Here's how the part is built. I have some questions about the finished solid (model axes, mm). A direction names the side the tool comes from. Round coordinates to 2 decimals unless told otherwise and drop trailing zeros. Write each loop counter-clockwise with the first axis right and the second up, starting at its lowest first coordinate (ties: lowest second). Pieces come first, ordered by that corner, then holes. Notation, with made-up numbers: M 41.5,38.5 L 65.5,38.5 A21 cw 65.5,42.5 Z; hole C 79,89.25 d4. An arc over 180 degrees is marked long. Write item = value, one per line. Start each with the question number.
(1) I want a section at C-C (z = -33). List the corners of the cut face in (x, y) for me.
(2) On a 3-axis mill with a long thin cutter (end or side, diameter ignored), from which of +Z, -Z, +X, -X, +Y, -Y can I reach the whole of each face in a straight line? I mean faces 1 (the flat face through (140, 2, -77)), 2 (the flat face through (98, 0, -24)), 3 (the flat face through (146.216, 1.972, 46.336)), 4 (the flat face through (160, 2, -73)), 5 (the flat face through (49.06, 1.97, 44.46)). Say none if no direction works.
(3) I want a section at D-D (y = 2.15). Give the number of separate pieces and of enclosed holes in the cut face, and give its area (3 significant figures).
(4) If we mould it in two halves opening along X, with no side actions, what happens to faces 6 (the flat face through (-4, 2, -9)), 7 (the flat face through (199, 2, 0)), 8 (the flat face through (190, 2, -75)), 9 (the cylindrical face through (100, 2, 62))? For each: released by +X, released by -X, zero draft, split by the parting line, or undercut.
(5) I want a section at A-A (z = -56). List the corners of the cut face in (x, y) for me, and give its area (3 significant figures).
(6) I want a section at B-B (x = 63). List the corners of the cut face in (y, z) for me.
(7) I need wall thicknesses on line 1 along X through (y, z) = (1.05, -33); line 2 along X through (y, z) = (2.8, -11.5); line 3 along X through (y, z) = (0.4, -53.5). Which ranges of each line are inside material? Lowest first, please.
(8) Will these pins go through, and if not, where does the flat tip stop? pin 1 Ø2 at (y, z) = (1.5, -74.5) entering from +X; pin 2 Ø1.5 at (x, y) = (152.5, 1) entering from -Z; pin 3 Ø2.5 at (x, z) = (137, -33) entering from -Y; pin 4 Ø1.5 at (x, y) = (97.5, 0.5) entering from -Z.
```python
from build123d import *

# Parameters (mm, degrees)
SKICA1_W                = 4
SKICA1_H                = 15
SKICA1_R                = 2.25
P_IDAT_VYSUNUT_M1_DEPTH = 4


with BuildPart() as part:
    # Skica1 → Přidat vysunutím1 (new body)
    with BuildSketch(Plane(origin=(0, 0, 0), x_dir=(1, 0, 0), z_dir=(0, 1, 0))):
        with BuildLine():
            ThreePointArc((10.915770195, 0), (25.940686176, -26.499731394), (48.580654593, -46.881480444))
            Line((48.580654593, -46.881480444), (49.547625125, -41.975874672))
            Line((49.547625125, -41.975874672), (54.453230897, -42.942845204))
            Line((54.453230897, -42.942845204), (53.134056197, -49.635242551))
            ThreePointArc((53.134056197, -49.635242551), (64.622092485, -55.166907964), (76.747418364, -59.110354723))
            Line((76.747418364, -59.110354723), (78.981259757, -47.777697862))
            Line((78.981259757, -47.777697862), (83.886865529, -48.744668394))
            Line((83.886865529, -48.744668394), (81.627559896, -60.206509669))
            ThreePointArc((81.627559896, -60.206509669), (100, -62), (118.372440104, -60.206509669))
            Line((118.372440104, -60.206509669), (116.113134471, -48.744668394))
            Line((116.113134471, -48.744668394), (121.018740243, -47.777697862))
            Line((121.018740243, -47.777697862), (123.252581636, -59.110354723))
            ThreePointArc((123.252581636, -59.110354723), (135.377907515, -55.166907964), (146.865943803, -49.635242551))
            Line((146.865943803, -49.635242551), (145.546769103, -42.942845204))
            Line((145.546769103, -42.942845204), (150.452374875, -41.975874672))
            Line((150.452374875, -41.975874672), (151.419345407, -46.881480444))
            ThreePointArc((151.419345407, -46.881480444), (174.059313824, -26.499731394), (189.084229805, 0))
            Line((189.084229805, 0), (209, 0))
            Line((209, 0), (209, 53))
            Line((209, 53), (200, 53))
            Line((200, 53), (200, 73))
            Line((200, 73), (190, 73))
            Line((190, 73), (190, 77))
            Line((190, 77), (170, 77))
            Line((170, 77), (170, 73))
            Line((170, 73), (150, 73))
            Line((150, 73), (150, 77))
            Line((150, 77), (130, 77))
            Line((130, 77), (130, 73))
            Line((130, 73), (115, 73))
            Line((115, 73), (115, 53))
            Line((115, 53), (85, 53))
            Line((85, 53), (85, 73))
            Line((85, 73), (70, 73))
            Line((70, 73), (70, 77))
            Line((70, 77), (50, 77))
            Line((50, 77), (50, 73))
            Line((50, 73), (30, 73))
            Line((30, 73), (30, 77))
            Line((30, 77), (10, 77))
            Line((10, 77), (10, 73))
            Line((10, 73), (0, 73))
            Line((0, 73), (0, 53))
            Line((0, 53), (-9, 53))
            Line((-9, 53), (-9, 0))
            Line((-9, 0), (10.915770195, 0))
        make_face()
        with Locations((-2, 9.5)):
            Rectangle(SKICA1_W, SKICA1_H, mode=Mode.SUBTRACT)
        with Locations((73.837049096, 6.837049096)):
            Circle(SKICA1_R, mode=Mode.SUBTRACT)
        with Locations((100, -4)):
            Circle(SKICA1_R, mode=Mode.SUBTRACT)
        with Locations((126.162950904, 6.837049096)):
            Circle(SKICA1_R, mode=Mode.SUBTRACT)
        with Locations((202, 9.5)):
            Rectangle(SKICA1_W, SKICA1_H, mode=Mode.SUBTRACT)
        with Locations((63, 33)):
            Circle(SKICA1_R, mode=Mode.SUBTRACT)
        with Locations((137, 33)):
            Circle(SKICA1_R, mode=Mode.SUBTRACT)
    extrude(amount=P_IDAT_VYSUNUT_M1_DEPTH)


solid = part.part
```
Returned:
q1.outline = M -9,0 L 60.75,0 L 60.75,4 L -9,4 Z; M 65.25,0 L 134.75,0 L 134.75,4 L 65.25,4 Z; M 139.25,0 L 209,0 L 209,4 L 139.25,4 Z
q2.face_1 = -Z, +X, -X, +Y, -Y
q2.face_2 = +Z, -Z, +X, -X, -Y
q2.face_3 = +Y, -Y
q2.face_4 = -Z, +Y, -Y
q2.face_5 = +Z, +Y, -Y
q3.separate_pieces = 1
q3.enclosed_holes = 7
q3.area = 22,900 mm²
q4.face_6 = undercut
q4.face_7 = zero draft
q4.face_8 = released by +X
q4.face_9 = split by the parting line
q5.outline = M 0,0 L 85,0 L 85,4 L 0,4 Z; M 115,0 L 200,0 L 200,4 L 115,4 Z
q5.area = 680 mm²
q6.outline = M 0,-77 L 4,-77 L 4,-35.25 L 0,-35.25 Z; M 0,-30.75 L 4,-30.75 L 4,54.5 L 0,54.5 Z
q7.line_1 = -9 to 60.75, 65.25 to 134.75, 139.25 to 209
q7.line_2 = -9 to -4, 0 to 200, 204 to 209
q7.line_3 = 0 to 85, 115 to 200
q8.pin_1 = 190
q8.pin_2 = -73
q8.pin_3 = through
q8.pin_4 = -53
